```python
from build123d import *

# Parameters (mm, degrees)
SKETCH1_R           = 2
BOSS_EXTRUDE1_DEPTH = 1.6
SKETCH1_3_W         = 8.2
SKETCH1_3_H         = 8.2
SKETCH1_3_W_2       = 6.2
SKETCH1_3_H_2       = 6.2
BOSS_EXTRUDE2_DEPTH = 2
BOSS_EXTRUDE3_START = -0.5
SKETCH1_4_W         = 8.2
SKETCH1_4_H         = 8.2
SKETCH1_4_W_2       = 6.2
SKETCH1_4_H_2       = 6.2
SKETCH1_4_R         = 2
BOSS_EXTRUDE3_DEPTH = 0.5
SKETCH3_W           = 5.8
SKETCH3_H           = 5.8
BOSS_EXTRUDE4_DEPTH = 4.5
CHAMFER1_SIZE       = 0.5
CUT_EXTRUDE1_DEPTH  = 0.2


with BuildPart() as part:
    # Sketch1 → Boss-Extrude1 (new body)
    with BuildSketch(Plane(origin=(0, 0, 0), x_dir=(1, 0, 0), z_dir=(0, 1, 0))):
        with Locations(Location((0, 0, 0), (0, 0, 270))):
            Circle(SKETCH1_R)
    extrude(amount=BOSS_EXTRUDE1_DEPTH)



with BuildPart() as body_2:
    # Sketch1_3 → Boss-Extrude2 (new body)
    with BuildSketch(Plane(origin=(0, 0, 0), x_dir=(1, 0, 0), z_dir=(0, 1, 0))):
        Rectangle(SKETCH1_3_W, SKETCH1_3_H)
        Rectangle(SKETCH1_3_W_2, SKETCH1_3_H_2, mode=Mode.SUBTRACT)
    extrude(amount=BOSS_EXTRUDE2_DEPTH)


with BuildPart() as part_1:
    add(part.part)

    add(body_2.part)  # Boss-Extrude3 merges body 2
    # Sketch1_4 → Boss-Extrude3 (add)
    # profile 1 of 3: a face of its own
    with BuildSketch(Plane(origin=(0, 0, 0), x_dir=(1, 0, 0), z_dir=(0, 1, 0)).offset(BOSS_EXTRUDE3_START)):
        Rectangle(SKETCH1_4_W, SKETCH1_4_H)
        Rectangle(SKETCH1_4_W_2, SKETCH1_4_H_2, mode=Mode.SUBTRACT)
    # profile 2 of 3: a face of its own
    with BuildSketch(Plane(origin=(0, 0, 0), x_dir=(1, 0, 0), z_dir=(0, 1, 0)).offset(BOSS_EXTRUDE3_START)):
        Rectangle(SKETCH1_4_W_2, SKETCH1_4_H_2)
        with Locations(Location((0, 0, 0), (0, 0, 270))):
            Circle(SKETCH1_4_R, mode=Mode.SUBTRACT)
    # profile 3 of 3: a face of its own
    with BuildSketch(Plane(origin=(0, 0, 0), x_dir=(1, 0, 0), z_dir=(0, 1, 0)).offset(BOSS_EXTRUDE3_START)):
        with Locations(Location((0, 0, 0), (0, 0, 270))):
            Circle(SKETCH1_4_R)
    extrude(amount=BOSS_EXTRUDE3_DEPTH)

    # Sketch3 → Boss-Extrude4 (add)
    with BuildSketch(Plane.XZ.offset(0.5)):
        Rectangle(SKETCH3_W, SKETCH3_H)
    extrude(amount=BOSS_EXTRUDE4_DEPTH)

    # Chamfer1
    chamfer1_edges = [part_1.edges().sort_by_distance(p)[0] for p in [
        (2.9, -2.75, -2.9),
        (2.9, -2.75, 2.9),
        (-2.9, -2.75, 2.9),
        (-2.9, -2.75, -2.9),
        (-4.1, 0.75, -4.1),
        (4.1, 0.75, -4.1),
        (4.1, 0.75, 4.1),
        (-4.1, 0.75, 4.1),
    ]]
    chamfer(chamfer1_edges, length=CHAMFER1_SIZE)

    # Sketch4 → Cut-Extrude1 (cut)
    with BuildSketch(Plane.XZ.offset(5)):
        with BuildLine():
            Line((-1.178429818, -1.660582309), (-1.178429818, 1.839417691))
            Line((-1.178429818, 1.839417691), (-0.471699048, 1.839417691))
            add(Edge.make_bspline(
                [(-0.471699048, 1.839417691), (-0.41023006, 1.838975121), (-0.291472295, 1.838120078), (-0.119859847, 1.832698686), (0.038923915, 1.823108221), (0.184356774, 1.809138694), (0.316837986, 1.791985661), (0.435996594, 1.770485257), (0.542448737, 1.745097086), (0.607918178, 1.723451636), (0.638877875, 1.713215767)],
                knots=[0, 0, 0, 0, 1.314313732, 2.53924729, 3.670748893, 4.714932338, 5.66265055, 6.526160246, 7.303039223, 8, 8, 8, 8], degree=3))
            add(Edge.make_bspline(
                [(0.638877875, 1.713215767), (0.679372614, 1.697785062), (0.759443806, 1.667273568), (0.873450929, 1.609717266), (0.980776292, 1.544504165), (1.081995437, 1.471548302), (1.174796263, 1.388783953), (1.26280416, 1.299726868), (1.342418884, 1.201138528), (1.41532718, 1.09506354), (1.481062839, 0.982751487), (1.538201997, 0.864416379), (1.58565599, 0.740659171), (1.625049217, 0.611824023), (1.656095674, 0.477627645), (1.677277606, 0.337913779), (1.691248596, 0.193234589), (1.692652647, 0.095060126), (1.693365054, 0.045247017)],
                knots=[0, 0, 0, 0, 0.984719456, 1.947108742, 2.898477687, 3.838006223, 4.779231079, 5.722358779, 6.681677486, 7.655904652, 8.64651281, 9.637519902, 10.640069247, 11.656948941, 12.698408672, 13.768548281, 14.867775369, 16, 16, 16, 16], degree=3))
            add(Edge.make_bspline(
                [(1.693365054, 0.045247017), (1.692736087, 0.001985779), (1.691496641, -0.08326501), (1.680367325, -0.208905906), (1.664191005, -0.330819477), (1.639146807, -0.448425177), (1.608744293, -0.562753395), (1.569780142, -0.672585639), (1.525144646, -0.778929449), (1.473094767, -0.880346924), (1.415953382, -0.976430297), (1.354631639, -1.067005825), (1.289194944, -1.150781047), (1.219019311, -1.228009659), (1.145011594, -1.298575237), (1.066687264, -1.363067252), (0.983844213, -1.420223807), (0.89685349, -1.472290916), (0.803177361, -1.517711271), (0.701041495, -1.556141281), (0.590010317, -1.587987896), (0.47035636, -1.614558792), (0.341872882, -1.635636095), (0.204433916, -1.649762487), (0.058250627, -1.65931542), (-0.042128638, -1.660151813), (-0.093794401, -1.660582309)],
                knots=[0, 0, 0, 0, 1.105936401, 2.179363191, 3.223086493, 4.248585256, 5.251745608, 6.245858792, 7.225916811, 8.198733463, 9.158002045, 10.082870192, 10.993790845, 11.873723703, 12.748670949, 13.606408763, 14.465103618, 15.319838547, 16.196477973, 17.123216899, 18.106603292, 19.147568657, 20.255746949, 21.433717677, 22.679120308, 24, 24, 24, 24], degree=3))
            Line((-0.093794401, -1.660582309), (-1.178429818, -1.660582309))
        make_face()
        with BuildLine():
            Line((-0.864327254, -1.30160795), (-0.462584465, -1.30160795))
            add(Edge.make_bspline(
                [(-0.462584465, -1.30160795), (-0.404856094, -1.301359854), (-0.293823296, -1.300882674), (-0.134165299, -1.296695471), (0.011714098, -1.289853533), (0.143835607, -1.280278455), (0.262124632, -1.26760984), (0.366828381, -1.253484938), (0.45760364, -1.235887487), (0.512533077, -1.219936527), (0.537916336, -1.212565483)],
                knots=[0, 0, 0, 0, 1.375205317, 2.645023457, 3.804390687, 4.853969522, 5.800190428, 6.637939096, 7.370582563, 8, 8, 8, 8], degree=3))
            add(Edge.make_bspline(
                [(0.537916336, -1.212565483), (0.569864698, -1.201313924), (0.632998337, -1.179079551), (0.723879422, -1.13852189), (0.808636426, -1.09047982), (0.888746452, -1.037077546), (0.963073107, -0.976431544), (1.032497223, -0.909860555), (1.096879025, -0.83702578), (1.155553333, -0.758017619), (1.208061637, -0.673327823), (1.253532866, -0.583788989), (1.293384398, -0.490382179), (1.32466299, -0.39167302), (1.349178575, -0.288543962), (1.366543263, -0.180987749), (1.377357987, -0.069024467), (1.378619435, 0.007127657), (1.37926249, 0.045948139)],
                knots=[0, 0, 0, 0, 0.998632004, 1.973411704, 2.929992603, 3.868527914, 4.809262121, 5.754881198, 6.702106254, 7.672490631, 8.653608572, 9.636854334, 10.631411391, 11.644891563, 12.686317036, 13.754757253, 14.855430412, 16, 16, 16, 16], degree=3))
            add(Edge.make_bspline(
                [(1.37926249, 0.045948139), (1.378749203, 0.08688162), (1.377740845, 0.167295804), (1.365066535, 0.285286499), (1.346544979, 0.39876715), (1.319761293, 0.507745345), (1.285630414, 0.612433697), (1.243035773, 0.712253207), (1.194369153, 0.808258076), (1.136465816, 0.898232442), (1.073050223, 0.983325551), (1.002672344, 1.061280467), (0.926450305, 1.132274767), (0.845215456, 1.19741408), (0.756678357, 1.254077756), (0.662924666, 1.304764437), (0.562578995, 1.347780328), (0.492766299, 1.370659191), (0.45728733, 1.38228628)],
                knots=[0, 0, 0, 0, 1.122418816, 2.205001699, 3.251619955, 4.274784885, 5.280384055, 6.268708349, 7.249350384, 8.229342522, 9.199999885, 10.157847722, 11.105861043, 12.055065948, 13.010012805, 13.98527497, 14.976112212, 16, 16, 16, 16], degree=3))
            add(Edge.make_bspline(
                [(0.45728733, 1.38228628), (0.427936183, 1.390402708), (0.365527593, 1.407660461), (0.263688129, 1.426485833), (0.14907298, 1.443090332), (0.021173279, 1.457148372), (-0.11986518, 1.467235693), (-0.274150868, 1.474807008), (-0.441750473, 1.47991364), (-0.557933007, 1.480262347), (-0.618233504, 1.480443332)],
                knots=[0, 0, 0, 0, 0.674548936, 1.434276114, 2.292660221, 3.240891867, 4.284742987, 5.42552168, 6.663806718, 8, 8, 8, 8], degree=3))
            Line((-0.618233504, 1.480443332), (-0.864327254, 1.480443332))
            Line((-0.864327254, 1.480443332), (-0.864327254, -1.30160795))
        make_face(mode=Mode.SUBTRACT)
    extrude(amount=-CUT_EXTRUDE1_DEPTH, mode=Mode.SUBTRACT)


solid = part_1.part
```
Input: part model. Units: mm. Frame: model coordinates. A direction names the side the tool comes from. Give positions to 0.01 mm unless a question says otherwise; leave off trailing zeros. Order: outer loops, then holes, each group sorted by start corner. A loop starts at its lowest first (then second) coordinate and runs counter-clockwise, first axis right, second up. Notation, with made-up numbers: (73.5, -24) - (115.5, -24) arc R20 ccw to (115.5, -20) - close; hole circle Ø3 at (-16.5, 62). An arc over 180 degrees is marked (long way). One line per item, written item: value.
1. Pin query (flat end, axial travel): pin 1 Ø1.3 at (y, z) = (-3.5, -1) entering from -X; pin 2 Ø3 at (x, z) = (-0.5, -0.5) entering from +Y; pin 3 Ø2 at (x, y) = (0, -3) entering from -Z. Return the tip coordinate at first contact, or that it passes through.
Determined:
pin 1: x = -2.9
pin 2: y = 1.6
pin 3: z = -2.9
2. Cut plane A-A, the plane y = 0.75. Output: boundary loops of the cut face in (x, z), and give its area (3 significant figures).
Determined:
outline: (-4.1, -3.6) - (-3.6, -4.1) - (3.6, -4.1) - (4.1, -3.6) - (4.1, 3.6) - (3.6, 4.1) - (-3.6, 4.1) - (-4.1, 3.6) - close; circle Ø4 at (0, 0); hole (-3.1, -3.1) - (3.1, -3.1) - (3.1, 3.1) - (-3.1, 3.1) - close
area: 40.9 mm2
3. Cut plane B-B, the plane y = -2.75. Output: boundary loops of the cut face in (x, z).
Determined:
outline: (-2.9, -2.4) - (-2.4, -2.9) - (2.4, -2.9) - (2.9, -2.4) - (2.9, 2.4) - (2.4, 2.9) - (-2.4, 2.9) - (-2.9, 2.4) - close
4. Cut plane C-C, the plane x = 2.75. Output: boundary loops of the cut face in (y, z).
Determined:
outline: (-5, -2.55) - (-0.5, -2.55) - (-0.5, -4.1) - (2, -4.1) - (2, -3.1) - (0, -3.1) - (0, 3.1) - (2, 3.1) - (2, 4.1) - (-0.5, 4.1) - (-0.5, 2.55) - (-5, 2.55) - close
5. Draft query along Z for faces 4 (the face through (0, -3, -2.9)), 5 (the face through (3.1, 1, 0)), 6 (the face through (4.1, 1, 0)). Return one class per face: released by +Z, released by -Z, zero draft, split by the parting line, or undercut.
Determined:
face 4: released by -Z
face 5: undercut
face 6: zero draft
6. Reachability of faces 1 (the face through (-2, 1, 0)), 2 (the face through (2.9, -3, 0)), 3 (the face through (-3.7, -0.5, -0.1)) from +Z, -Z, +X, -X, +Y, -Y: full face, straight path, thin tool, end or side. Return the list, or none.
Determined:
face 1: +Y
face 2: +Z, -Z, +X, -Y
face 3: -Y
7. Line query: probe 1 along Z at (x, y) = (-1, 0.5); probe 2 along Z at (x, y) = (-1.5, 0.25); probe 3 along Z at (x, y) = (-2.5, 1.5). Output: solid intervals per line, ascending.
Determined:
probe 1: -4.1 to -3.1, -1.73 to 1.73, 3.1 to 4.1
probe 2: -4.1 to -3.1, -1.32 to 1.32, 3.1 to 4.1
probe 3: -4.1 to -3.1, 3.1 to 4.1
